from build123d import *

# Parameters (mm, degrees)
SKETCH1_R           = 2.54
BOSS_EXTRUDE1_DEPTH = 2.54
SKETCH2_W           = 38.1
SKETCH2_H           = 12.7
BOSS_EXTRUDE2_DEPTH = 2.54
FILLET1_R           = 1.27


with BuildPart() as part:
    # Sketch1 → Boss-Extrude1 (new body)
    with BuildSketch(Plane.XY):
        with BuildLine():
            Line((-54.601784234, -110.868808086), (-21.972951858, -21.22182791))
            ThreePointArc((-21.972951858, -21.22182791), (-25.76817209, -13.082951858), (-33.907048142, -16.87817209))
            Line((-33.907048142, -16.87817209), (-66.918832376, -107.577303848))
            ThreePointArc((-66.918832376, -107.577303848), (-67.205313465, -108.64646583), (-67.301784234, -109.749131758))
            Line((-67.301784234, -109.749131758), (-67.301784234, -162.56))
            Line((-67.301784234, -162.56), (-80.001784234, -162.56))
            Line((-80.001784234, -162.56), (-80.001784234, -175.26))
            Line((-80.001784234, -175.26), (-41.901784234, -175.26))
            Line((-41.901784234, -175.26), (-41.901784234, -162.56))
            Line((-41.901784234, -162.56), (-54.601784234, -162.56))
            Line((-54.601784234, -162.56), (-54.601784234, -110.868808086))
        make_face()
        with Locations((-27.94, -19.05)):
            Circle(SKETCH1_R, mode=Mode.SUBTRACT)
        with Locations((-60.951784234, -109.749131758)):
            Circle(SKETCH1_R, mode=Mode.SUBTRACT)
    extrude(amount=BOSS_EXTRUDE1_DEPTH)

    # Sketch2 → Boss-Extrude2 (add)
    with BuildSketch(Plane(origin=(0, 0, 0), x_dir=(-1, 0, 0), z_dir=(0, 0, -1))):
        with Locations((60.951784234, -168.91)):
            Rectangle(SKETCH2_W, SKETCH2_H)
    extrude(amount=BOSS_EXTRUDE2_DEPTH)

    # Fillet1
    fillet1_edges = [part.edges().sort_by_distance(p)[0] for p in [
        (-54.601784234, -162.56, 1.27),
        (-67.301784234, -162.56, 1.27),
        (-60.951784234, -162.56, 0),
    ]]
    fillet(fillet1_edges, radius=FILLET1_R)


solid = part.part
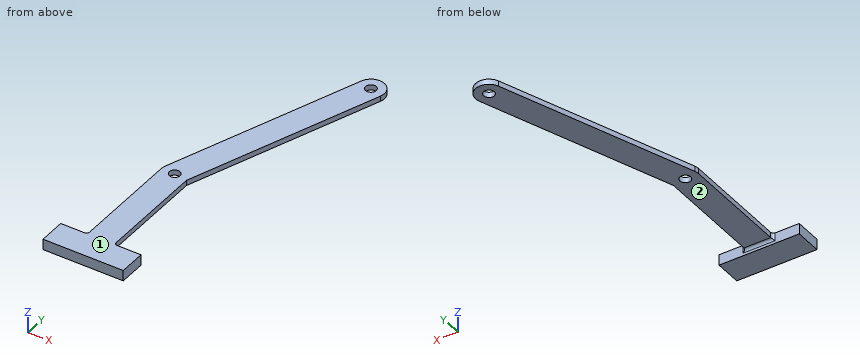
Source: CAD feature listing. Evaluate the final solid. Frame: model axes, mm. Face numbers are marked on the shaded views. A direction names the side the tool comes from. Coordinates: 2 decimals unless noted, no trailing zeros. Loops run counter-clockwise (first coordinate to the right, second up) from the corner with the lowest first, then second, coordinate; pieces in that order, holes last. Notation, with made-up numbers: (29.5, -9.75) - (63.5, -9.75) arc R27 ccw to (63.5, 17.25) - close; hole circle Ø3 at (-4, 27). An arc over 180 degrees is marked (long way). One line per item, written item: value. Start each with the question number.
1. Section C-C (x = -57). Return the cut outline in (y, z).
2. Set-up query: the marked faces 1 and 2. Return all of +Z, -Z, +X, -X, +Y, -Y with unobstructed straight access to the full face (end or side cutting, diameter ignored); none if empty.
3. Ray query, L1, parallel to Y at x = -69, z = 0.6; L2, parallel to X at y = -118, z = 1.2; L3, parallel to Z at x = -57, y = -95.5. Return the intervals inside material, ascending.
4. Contact query for flat-ended pins moving along their axis: P1, Ø1.3, axis at y = -134.5, z = 0.5, coming from the +X side; P2, Ø4.5, axis at x = -60.95, y = -109.75, coming from the +Z side; P3, Ø2.5, axis at y = -168.5, z = -1, coming from the +X side; P4, Ø3, axis at y = -141, z = 1.5, coming from the -X side. Output: stop coordinate, or through.
5. Section B-B (y = -19.05). Return the cut outline in (x, z), and give its area (3 significant figures).
6. Section D-D (y = -125.5). Return the cut outline in (x, z).
7. Section A-A (x = -27.94). Return the cut outline in (y, z), and give its area (3 significant figures).
Verdict:
1. outline: (-175.26, -2.54) - (-162.56, -2.54) - (-162.56, -1.27) arc R1.27 cw to (-161.29, 0) - (-80.33, 0) - (-80.33, 2.54) - (-175.26, 2.54) - close
2. face 1: +Z, +X, -X, +Y, -Y
2. face 2: -Z, +X, -X, +Y
3. L1: y = -175.26 to -162.56
3. L2: x = -67.3 to -54.6
3. L3: z = 0 to 2.54
4. P1: stops at x = -54.6
4. P2: passes through
4. P3: stops at x = -41.9
4. P4: stops at x = -67.3
5. outline: (-34.7, 0) - (-30.48, 0) - (-30.48, 2.54) - (-34.7, 2.54) - close; (-25.4, 0) - (-21.59, 0) - (-21.59, 2.54) - (-25.4, 2.54) - close
5. area: 20.4 mm2
6. outline: (-67.3, 0) - (-54.6, 0) - (-54.6, 2.54) - (-67.3, 2.54) - close
7. outline: (-37.62, 0) - (-21.59, 0) - (-21.59, 2.54) - (-37.62, 2.54) - close; (-16.51, 0) - (-12.7, 0) - (-12.7, 2.54) - (-16.51, 2.54) - close
7. area: 50.4 mm2
